```python
from build123d import *

# Parameters (mm, degrees)
SKETCH1_R                = 17
BOSS_EXTRUDE1_DEPTH      = 3
SKETCH3_R                = 17
BOSS_EXTRUDE2_DEPTH      = 3
BOSS_EXTRUDE3_DEPTH      = 31
CUT_EXTRUDE11_DEPTH      = 60
CUT_EXTRUDE11_DEPTH_BACK = 50
SKETCH7_R                = 1.751351815
CUT_EXTRUDE1_DEPTH       = 50
SKETCH8_W                = 7.5
SKETCH8_H                = 2
CUT_EXTRUDE12_DEPTH      = 30
SKETCH9_R                = 19.5
SKETCH9_R_2              = 18
BOSS_EXTRUDE4_DEPTH      = 38
FILLET1_R                = 2
SKETCH10_R               = 19.500000009
SKETCH10_R_2             = 17.00000001
BOSS_EXTRUDE5_DEPTH      = 3


with BuildPart() as part:
    # Sketch1 → Boss-Extrude1 (new body)
    with BuildSketch(Plane(origin=(0, -15, 0), x_dir=(1, 0, 0), z_dir=(0, 1, 0))):
        with Locations(Location((0, 0, 0), (0, 0, 270))):
            Circle(SKETCH1_R)
    extrude(amount=BOSS_EXTRUDE1_DEPTH)



with BuildPart() as body_2:
    # Sketch3 → Boss-Extrude2 (new body)
    with BuildSketch(Plane(origin=(0, 21, 0), x_dir=(1, 0, 0), z_dir=(0, 1, 0))):
        with Locations(Location((0, 0, 0), (0, 0, 270))):
            Circle(SKETCH3_R)
    extrude(amount=-BOSS_EXTRUDE2_DEPTH)


with BuildPart() as part_1:
    add(part.part)

    add(body_2.part)  # Boss-Extrude3 merges body 2
    # Sketch6 → Boss-Extrude3 (add)
    with BuildSketch(Plane(origin=(0, -12, 0), x_dir=(1, 0, 0), z_dir=(0, 1, 0))):
        Polygon((-10.39609313, -6.860559341), (-11.68775931, -8.152225055), (-12.244775891, -7.288892753), (-12.738139369, -6.387668662), (-13.165283017, -5.453239195), (-13.523988426, -4.490460269), (-13.812389225, -3.504338907), (-14.028987847, -2.499999944), (-12.202296406, -2.499999944), (-12.202296406, 2.499999944), (-14.028987847, 2.499999944), (-13.812389225, 3.504338907), (-13.523988426, 4.490460269), (-13.165283017, 5.453239195), (-12.738139369, 6.387668662), (-12.244775891, 7.288892753), (-11.68775931, 8.152225055), (-10.39609313, 6.860559341), (-6.860559341, 10.39609313), (-8.152225055, 11.68775931), (-7.288892753, 12.244775891), (-6.387668662, 12.738139369), (-5.453239195, 13.165283017), (-4.490460269, 13.523988426), (-3.504338907, 13.812389225), (-2.499999944, 14.028987847), (-2.499999944, 12.174172863), (2.499999944, 12.202296406), (2.499999944, 14.028987847), (3.504338907, 13.812389225), (4.490460269, 13.523988426), (5.453239195, 13.165283017), (6.387668662, 12.738139369), (7.288892753, 12.244775891), (8.152225055, 11.68775931), (6.860559341, 10.39609313), (10.39609313, 6.860559341), (11.68775931, 8.152225055), (12.244775891, 7.288892753), (12.738139369, 6.387668662), (13.165283017, 5.453239195), (13.523988426, 4.490460269), (13.812389225, 3.504338907), (14.028987847, 2.499999944), (12.202296406, 2.499999944), (12.202296406, -2.499999944), (14.028987847, -2.499999944), (13.812389225, -3.504338907), (13.523988426, -4.490460269), (13.165283017, -5.453239195), (12.738139369, -6.387668662), (12.244775891, -7.288892753), (11.68775931, -8.152225055), (10.39609313, -6.860559341), (6.860559341, -10.39609313), (8.152225055, -11.68775931), (7.288892753, -12.244775891), (6.387668662, -12.738139369), (5.453239195, -13.165283017), (4.490460269, -13.523988426), (3.504338907, -13.812389225), (2.499999944, -14.028987847), (2.499999944, -12.202296406), (-2.499999944, -12.202296406), (-2.499999944, -14.028987847), (-3.504338907, -13.812389225), (-4.490460269, -13.523988426), (-5.453239195, -13.165283017), (-6.387668662, -12.738139369), (-7.288892753, -12.244775891), (-8.152225055, -11.68775931), (-6.860559341, -10.39609313), align=None)
    extrude(amount=BOSS_EXTRUDE3_DEPTH)

    # Sketch7 → Cut-Extrude11 (cut, two sides: drawn at the far end of the back side and taken through both)
    with BuildSketch(Plane(origin=(-0.068553102, 0, -12.187849043), x_dir=(-0.9999841817006155, 0, 0.005624619858302935), z_dir=(-0.005624619858302935, 0, -0.9999841817006155)).offset(-CUT_EXTRUDE11_DEPTH_BACK)):
        with Locations(Location((-0.120761258, 1.306302196, 0), (0, 0, 180))):
            Circle(SKETCH7_R)
    extrude(amount=CUT_EXTRUDE11_DEPTH + CUT_EXTRUDE11_DEPTH_BACK, mode=Mode.SUBTRACT)

    # Sketch2 → Cut-Extrude1 (cut)
    with BuildSketch(Plane(origin=(0, -15, 0), x_dir=(1, 0, 0), z_dir=(0, 1, 0))):
        with BuildLine():
            Line((2.642344683, 1.420568442), (-2.642344683, 1.420568442))
            ThreePointArc((-2.642344683, 1.420568442), (0, -2.999999869), (2.642344683, 1.420568442))
        make_face()
    extrude(amount=CUT_EXTRUDE1_DEPTH, mode=Mode.SUBTRACT)

    # Sketch8 → Cut-Extrude12 (cut)
    with BuildSketch(Plane(origin=(0, -15, 0), x_dir=(1, 0, 0), z_dir=(0, 1, 0))):
        with Locations((-0.237061367, 10.505385433)):
            Rectangle(SKETCH8_W, SKETCH8_H)
    cut_extrude12 = extrude(amount=CUT_EXTRUDE12_DEPTH, mode=Mode.SUBTRACT)

    # Mirror1: Cut-Extrude12 across plane
    add(cut_extrude12.mirror(Plane.XY), mode=Mode.SUBTRACT)



with BuildPart() as body_2_2:
    # Sketch9 → Boss-Extrude4 (new body)
    with BuildSketch(Plane(origin=(0, -15, 0), x_dir=(1, 0, 0), z_dir=(0, 1, 0))):
        with Locations(Location((0, 0, 0), (0, 0, 270))):
            Circle(SKETCH9_R)
        with Locations(Location((0, 0, 0), (0, 0, 270))):
            Circle(SKETCH9_R_2, mode=Mode.SUBTRACT)
    extrude(amount=BOSS_EXTRUDE4_DEPTH)

    # Fillet1
    # the kernel refuses this fillet: 2 mm, written as the material it takes off along each edge
    with BuildSketch(Plane(origin=(0, 23, 0), x_dir=(0, 0, 1), z_dir=(-1, 0, 0))) as fillet1_piece_1:
        with BuildLine():
            CenterArc((20, -1.936491673), FILLET1_R, 104.477512186, 75.522487814)
            Line((19.5, 0), (19.49, 0.038729833))
            ThreePointArc((19.49, 0.038729833), (18.75, 0.04), (18, 0.04))
            Line((18, 0.04), (17.96, 0))
            Line((17.96, 0), (17.96, -1.936491673))
            Line((17.96, -1.936491673), (18, -1.936491673))
        make_face()
    revolve(axis=Axis((0, 23, 0), (0, 1, 0)), mode=Mode.SUBTRACT)


with BuildPart() as part_2:
    add(part_1.part)

    add(body_2_2.part)  # Boss-Extrude5 merges body 2 2
    # Sketch10 → Boss-Extrude5 (add)
    with BuildSketch(Plane(origin=(0, -15, 0), x_dir=(1, 0, 0), z_dir=(0, 1, 0))):
        with Locations(Location((0, 1.03e-07, 0), (0, 0, 270))):
            Circle(SKETCH10_R)
        with Locations(Location((0, 1.03e-07, 0), (0, 0, 270))):
            Circle(SKETCH10_R_2, mode=Mode.SUBTRACT)
    extrude(amount=BOSS_EXTRUDE5_DEPTH)


solid = part_2.part
```
Can you work these out from the model? Positions are in its coordinate system, mm. A direction names the side the tool comes from. Round coordinates to 2 decimals unless told otherwise and drop trailing zeros. Order: outer loops, then holes, each group sorted by start corner. A loop starts at its lowest first (then second) coordinate and runs counter-clockwise, first axis right, second up.
(1) On a 3-axis mill with a long thin cutter (end or side, diameter ignored), from which of +Z, -Z, +X, -X, +Y, -Y can I reach the whole of each face in a straight line? I mean faces 4 (the face through (-7.515, 2.79, 11.051)), 5 (the face through (-1.41, 2.75, 2.65)), 6 (the face through (-4, -15, 0)), 7 (the face through (16.855, 19.521, -2.213)), 8 (the face through (3.513, 0, -10)). Say none if no direction works.
Results are:
face 4: none
face 5: +Y, -Y
face 6: +Z, -Z, +X, -X, -Y
face 7: +Y
face 8: -Y
(2) We'd pull the mould along Y, two halves only. Please class faces 1 (the face through (0, 15, 11)), 2 (the face through (13, 3, -2.5)), 3 (the face through (-1.1, -0.2, -9.505)): +Y half, -Y half, draft (parallel to the pull), parting line (faces both ways), or undercut.
Results are:
face 1: -Y half
face 2: undercut
face 3: draft
(3) If we section it at A-A (z = 0): Please give me the cut outline in (x, y).
Results are:
outline: (-19.5, -15) - (-3, -15) - (-3, 21) - (-17, 21) - (-17, 18) - (-12.2, 18) - (-12.2, -12) - (-18, -12) - (-18, 21.06) arc R2 ccw to (-19.5, 23) - close; (3, -15) - (19.5, -15) - (19.5, 23) arc R2 ccw to (18, 21.06) - (18, -12) - (12.2, -12) - (12.2, 18) - (17, 18) - (17, 21) - (3, 21) - close
(4) I'm going to push flat-ended pins straight in: pin 1 (1.5 mm diameter, centred on y = 9.5, z = 13, fed in from +X); pin 2 (0.6 mm diameter, centred on y = -2.5, z = 10, fed in from -X); pin 3 (4 mm diameter, centred on x = -13, y = 4, fed in from +Z). Where does each tip first touch, or does it pass through?
Results are:
pin 1: stops at x = 15.17
pin 2: stops at x = -16.92
pin 3: stops at z = 16.1
(5) If we section it at B-B (y = -6.5): Count the separate pieces of the cut face and the enclosed holes in it, plus the area to 3 significant figures.
Results are:
separate pieces: 2
enclosed holes: 4
area: 683 mm2
(6) If I drill on L1, parallel to X at y = -4, z = 0; L2, parallel to Y at x = 9.5, z = -14; L3, parallel to Z at x = 4, y = 20, over which ranges is the centre line in solid material (lowest first)?
Results are:
L1: x = -19.5 to -18, -12.2 to -3, 3 to 12.2, 18 to 19.5
L2: y = -15 to -12, 18 to 21
L3: z = -19.09 to -17.55, -16.52 to 16.52, 17.55 to 19.09
